Verification items for the finished model (mm, model axes). A direction names the side the tool comes from. Round coordinates to 2 decimals unless told otherwise and drop trailing zeros. Order: outer loops, then holes, each group sorted by start corner. A loop starts at its lowest first (then second) coordinate and runs counter-clockwise, first axis right, second up. Notation, with made-up numbers: (23.5, -36) -> (66.5, -36) arc R12 cw to (66.5, -23) -> close; hole circle Ø6 at (85, 53.5). An arc over 180 degrees is marked (long way). Put each result on its own line as item: value.
from build123d import *

# Parameters (mm, degrees)
BOSS_EXTRUDE1_DEPTH = 600
BOSS_EXTRUDE2_DEPTH = 100


with BuildPart() as part:
    # Sketch1 → Boss-Extrude1 (new body)
    with BuildSketch(Plane.XY):
        Polygon((-65, 100), (65, 100), (60, 95.25), (45, 81), (-45, 81), (-60, 95.25), align=None)
    extrude(amount=-BOSS_EXTRUDE1_DEPTH)

    # Sketch2 → Boss-Extrude2 (add)
    with BuildSketch(Plane.XZ):
        Polygon((-45, -15), (-60, 0), (60, 0), (45, -15), align=None)
    extrude(amount=-BOSS_EXTRUDE2_DEPTH)


solid = part.part
Item 1: Section check A-A on x = -22.5. Record the boundary of the cut face in (y, z).
Check sheet entries:
outline: (0, -15) -> (81, -15) -> (81, -600) -> (100, -600) -> (100, 0) -> (0, 0) -> close
Item 2: Section check B-B on y = 53.5. Record the boundary of the cut face in (x, z), then the cut area to 4 significant figures.
Check sheet entries:
outline: (-60, 0) -> (-45, -15) -> (45, -15) -> (60, 0) -> close
area: 1,575 mm^2
Item 3: Tool access check on faces 1 (the flat face through (1, 40, -15)), 2 (the flat face through (-1, 100, -296)), 3 (the flat face through (53, 47, -7)), 4 (the flat face through (-1, 49, 0)), 5 (the flat face through (-52, 47, -8)). Record the directions out of +Z, -Z, +X, -X, +Y, -Y that give a thin tool (end or side, any length) a straight path to the whole face; none if there is none.
Check sheet entries:
face 1: -Z, +X, -X, -Y
face 2: +Z, -Z, +X, -X, +Y
face 3: -Z, +X, -Y
face 4: +Z, +X, -X, +Y, -Y
face 5: -Z, -X, -Y
Item 4: Gauge pin test, flat ends, axial feed: pin 1 Ø10 at (y, z) = (78.5, -520) entering from -X; pin 2 Ø8 at (x, z) = (-12, -90) entering from -Y; pin 3 Ø1.5 at (y, z) = (80.5, -108) entering from -X. Record the tip position at first contact, or that the pin passes through.
Check sheet entries:
pin 1: stops at x = -47.63
pin 2: stops at y = 81
pin 3: stops at x = -45.26
Item 5: Section check C-C on z = -265. Record the boundary of the cut face in (x, y).
Check sheet entries:
outline: (-65, 100) -> (-45, 81) -> (45, 81) -> (65, 100) -> close
Item 6: Material ranges on L1, parallel to Y at x = -37.5, z = -281; L2, parallel to Z at x = 28.5, y = 42; L3, parallel to X at y = 83, z = -304, recorded low to high. Write a range as [from, to].
Check sheet entries:
L1: y = [81, 100]
L2: z = [-15, 0]
L3: x = [-47.11, 47.11]
